Input: part model. Units: mm. Frame: model coordinates. A direction names the side the tool comes from. Give positions to 0.01 mm unless a question says otherwise; leave off trailing zeros. Loops run counter-clockwise (first coordinate to the right, second up) from the corner with the lowest first, then second, coordinate; pieces in that order, holes last. Notation, with made-up numbers: M 49.25,49 L 82.25,49 A24 ccw 82.25,88 Z; hole C -12.5,45.5 d3. An arc over 180 degrees is marked long. Answer as a JSON object with one key per item and string values. Group by question number.
```python
from build123d import *

# Parameters (mm, degrees)
SKETCH_1_W          = 36
SKETCH_1_H          = 48
LIFT_CARRIAGE_DEPTH = 36
FILLET_2_R          = 2
SKETCH_2_W          = 18
SKETCH_2_H          = 28
FRONT_RECESS_DEPTH  = 5
SKETCH_3_R          = 8.3
SCREW_PASSAGE_DEPTH = 70.971422738


with BuildPart() as part:
    # 草图1 → Lift_carriage (new body)
    with BuildSketch(Plane.XY):
        with Locations((18, 24)):
            Rectangle(SKETCH_1_W, SKETCH_1_H)
    extrude(amount=LIFT_CARRIAGE_DEPTH)

    # Fillet 2
    fillet_2_edges = [part.edges().sort_by_distance(p)[0] for p in [
        (36, 24, 36),
        (0, 24, 36),
        (36, 24, 0),
        (0, 24, 0),
    ]]
    fillet(fillet_2_edges, radius=FILLET_2_R)

    # 草图2 → Front_recess (cut)
    with BuildSketch(Plane.XY.offset(36)):
        with Locations((18, 21)):
            Rectangle(SKETCH_2_W, SKETCH_2_H)
    extrude(amount=-FRONT_RECESS_DEPTH, mode=Mode.SUBTRACT)

    # 草图3 → Screw_passage (cut, through all)
    with BuildSketch(Plane(origin=(0, 48, 0), x_dir=(1, 0, 0), z_dir=(0, 1, 0))):
        with Locations(Location((18, -18, 0), (0, 0, 270))):
            Circle(SKETCH_3_R)
    extrude(amount=-SCREW_PASSAGE_DEPTH, mode=Mode.SUBTRACT)


solid = part.part
```
1. Reachability of faces 4 (the cylindrical face through (12.95, 24.336, 11.413)), 5 (the flat face through (18, 7, 34)) from +Z, -Z, +X, -X, +Y, -Y: full face, straight path, thin tool, end or side. Return the list, or none.
2. Mould query, pull axis Y, two halves, no side actions, for faces 1 (the flat face through (26, 0, 22)), 2 (the cylindrical face through (0.57, 24.34, 35.4)), 3 (the flat face through (18, 35, 34)). Classes: pulls with the +Y half, pulls with the -Y half, needs draft (parallel to the pull), parting line crosses it, or undercut.
3. Section A-A (x = 18). Output: boundary loops of the cut face in (y, z), then the cut area to 3 significant figures.
4. Material intervals for L1, parallel to X at y = 28, z = 18; L2, parallel to Y at x = 16, z = 33; L3, parallel to X at y = 7.5, z = 31.5, sorted ascending.
5. Section B-B (y = 45.5). Output: boundary loops of the cut face in (x, z).
6. Section D-D (z = 11.5). Output: boundary loops of the cut face in (x, y).
7. Section C-C (z = 18). Output: boundary loops of the cut face in (x, y).
Geometry results:
{
 "1": {"face 4": "+Y, -Y", "face 5": "+Z"},
 "2": {"face 1": "pulls with the -Y half", "face 2": "needs draft", "face 3": "undercut"},
 "3": {"outline": "M 0,0 L 48,0 L 48,9.7 L 0,9.7 Z; M 0,26.3 L 48,26.3 L 48,36 L 35,36 L 35,31 L 7,31 L 7,36 L 0,36 Z", "area": "791 mm2"},
 "4": {"L1": "0 to 9.7, 26.3 to 36", "L2": "0 to 7, 35 to 48", "L3": "0 to 9, 27 to 36"},
 "5": {"outline": "M 0,2 A2 ccw 2,0 L 34,0 A2 ccw 36,2 L 36,34 A2 ccw 34,36 L 2,36 A2 ccw 0,34 Z; hole C 18,18 d16.6"},
 "6": {"outline": "M 0,0 L 12.84,0 L 12.84,48 L 0,48 Z; M 23.16,0 L 36,0 L 36,48 L 23.16,48 Z"},
 "7": {"outline": "M 0,0 L 9.7,0 L 9.7,48 L 0,48 Z; M 26.3,0 L 36,0 L 36,48 L 26.3,48 Z"}
}
